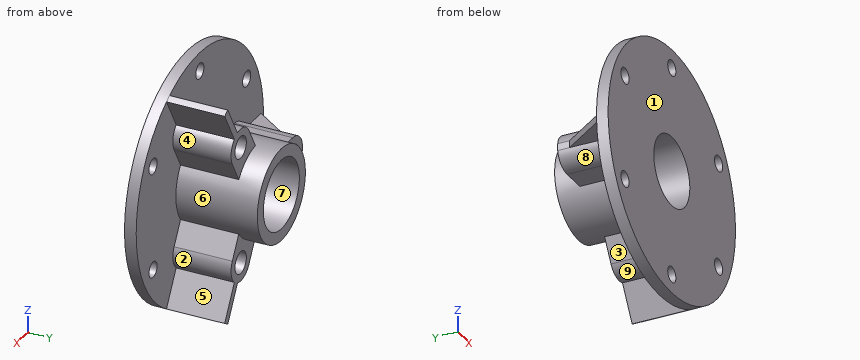
```python
from build123d import *
from build123d.topology import SkipClean

# Parameters (mm, degrees)
SKETCH1_R           = 53
BOSS_EXTRUDE1_DEPTH = 5
SKETCH2_R           = 20
BOSS_EXTRUDE2_DEPTH = 35
SKETCH3_R           = 15
CUT_EXTRUDE1_DEPTH  = 85.958813551
BOSS_EXTRUDE3_START = -25
SKETCH4_R           = 4.75
BOSS_EXTRUDE3_DEPTH = 25
CUT_EXTRUDE2_DEPTH  = 86.902561079
CIRPATTERN1_COUNT   = 3
SKETCH6_R           = 3.4
CUT_EXTRUDE3_DEPTH  = 83.722427431


with BuildPart() as part:
    # Sketch1 → Boss-Extrude1 (new body)
    with BuildSketch(Plane(origin=(0, 0, 0), x_dir=(1, 0, 0), z_dir=(0, 1, 0))):
        with Locations(Location((0, 0, 0), (0, 0, 270))):
            Circle(SKETCH1_R)
    extrude(amount=BOSS_EXTRUDE1_DEPTH)

    # Sketch2 → Boss-Extrude2 (add)
    with BuildSketch(Plane(origin=(0, 5, 0), x_dir=(1, 0, 0), z_dir=(0, 1, 0))):
        with Locations(Location((0, 0, 0), (0, 0, 270))):
            Circle(SKETCH2_R)
    extrude(amount=BOSS_EXTRUDE2_DEPTH)

    # Sketch3 → Cut-Extrude1 (cut, through all)
    with BuildSketch(Plane(origin=(0, 40, 0), x_dir=(1, 0, 0), z_dir=(0, 1, 0))):
        with Locations(Location((0, 0, 0), (0, 0, 270))):
            Circle(SKETCH3_R)
    extrude(amount=-CUT_EXTRUDE1_DEPTH, mode=Mode.SUBTRACT)

    # Sketch4 → Boss-Extrude3 (add)
    with BuildSketch(Plane(origin=(0, 30, 0), x_dir=(1, 0, 0), z_dir=(0, 1, 0)).offset(BOSS_EXTRUDE3_START)):
        with BuildLine():
            Line((-29, 8), (-18.33030278, 8))
            ThreePointArc((-18.33030278, 8), (-20, 0), (-18.33030278, -8))
            Line((-18.33030278, -8), (-29, -8))
            ThreePointArc((-29, -8), (-34.099019514, -6.164414003), (-36.858116823, -1.5))
            Line((-36.858116823, -1.5), (-52.978769333, -1.5))
            ThreePointArc((-52.978769333, -1.5), (-53, 0), (-52.978769333, 1.5))
            Line((-52.978769333, 1.5), (-36.858116823, 1.5))
            ThreePointArc((-36.858116823, 1.5), (-34.099019514, 6.164414003), (-29, 8))
        make_face()
        with Locations(Location((-29, 0, 0), (0, 0, 270))):
            Circle(SKETCH4_R, mode=Mode.SUBTRACT)
    boss_extrude3 = extrude(amount=BOSS_EXTRUDE3_DEPTH)

    # Sketch5 → Cut-Extrude2 (cut, through all)
    with BuildSketch(Plane.XY.offset(1.5)):
        Polygon((-36.858116823, 25), (-50.978769333, 5), (-53.978769333, 5), (-53.978769333, 30), (-36.858116823, 30), align=None)
    extrude(amount=-CUT_EXTRUDE2_DEPTH, mode=Mode.SUBTRACT)

    # CirPattern1: Boss-Extrude3 ×3 about axis
    with SkipClean():  # the faces are left unmerged after this step: merging them gives an invalid solid
        cirpattern1_axis = Axis((0, 0, 0), (0, 1, 0))
        for i in range(1, CIRPATTERN1_COUNT):
            add(boss_extrude3.rotate(cirpattern1_axis, i * 360 / CIRPATTERN1_COUNT))

    # Sketch6 → Cut-Extrude3 (cut, through all)
    with SkipClean():  # the faces are left unmerged after this step: merging them gives an invalid solid
        with BuildSketch(Plane(origin=(0, 5, 0), x_dir=(1, 0, 0), z_dir=(0, 1, 0))):
            with Locations(Location((0, 45, 0), (0, 0, 270))):
                Circle(SKETCH6_R)
            with Locations(Location((38.97114317, 22.5, 0), (0, 0, 270))):
                Circle(SKETCH6_R)
            with Locations(Location((38.97114317, -22.5, 0), (0, 0, 270))):
                Circle(SKETCH6_R)
            with Locations(Location((0, -45, 0), (0, 0, 270))):
                Circle(SKETCH6_R)
            with Locations(Location((-38.97114317, -22.5, 0), (0, 0, 270))):
                Circle(SKETCH6_R)
            with Locations(Location((-38.97114317, 22.5, 0), (0, 0, 270))):
                Circle(SKETCH6_R)
        extrude(amount=-CUT_EXTRUDE3_DEPTH, mode=Mode.SUBTRACT)


solid = part.part
```
Design review of the part built by this model. Coordinates are the model's own, in mm. Face numbers are marked on the shaded views. A direction names the side the tool comes from. Round coordinates to 2 decimals unless told otherwise and drop trailing zeros. Write each loop counter-clockwise with the first axis right and the second up, starting at its lowest first coordinate (ties: lowest second). Pieces come first, ordered by that corner, then holes.
Item 1: We need section D-D on y = 34.5. Write out the cut boundary in (x, z).
Item 2: We need section B-B on x = 0. Write out the cut boundary in (y, z).
Item 3: For probe 1 along X at (y, z) = (4, 20.5); probe 2 along X at (y, z) = (1, -22.5); probe 3 along Y at (x, z) = (-38.5, -10), list the stretches that pass through material, from the lowest coordinate up.
Item 4: We need section A-A on z = 0. Write out the cut boundary in (x, y), and give its area (3 significant figures).
Item 5: Clearance check with flat-ended pins moving along their axes: pin 1 Ø1.5 at (x, y) = (-5.5, 28) entering from -Z; pin 2 Ø3 at (x, y) = (-22.5, 17.5) entering from +Z; pin 3 Ø1.5 at (y, z) = (33.5, -9) entering from -X. State where each tip first meets the part, or that it passes through.
Item 6: The part is to be moulded in two halves that separate along Z. For the marked faces 1, 2, 3 and 4, say which applies: +Z half, -Z half, draft (parallel to the pull), parting line (faces both ways), or undercut.
Item 7: We need section C-C on y = 28.5. Write out the cut boundary in (x, z), and give its area (3 significant figures).
Item 8: For the marked faces 5, 6, 7, 8 and 9, list the 3-axis set-ups (+Z, -Z, +X, -X, +Y, -Y) from which the entire face can be reached by the end or side of a thin tool; tool diameter is ignored.
Returned:
1. outline: circle Ø40 at (0, 0); hole circle Ø30 at (0, 0)
2. outline: (0, -53) - (5, -53) - (5, -48.4) - (0, -48.4) - close; (0, -41.6) - (5, -41.6) - (5, -20) - (40, -20) - (40, -15) - (0, -15) - close; (0, 15) - (40, 15) - (40, 20) - (5, 20) - (5, 41.6) - (0, 41.6) - close; (0, 48.4) - (5, 48.4) - (5, 53) - (0, 53) - close
3. probe 1: x = -48.87 to -41.72, -36.22 to 36.22, 41.72 to 48.87
3. probe 2: x = -47.99 to -42.37, -35.57 to 35.57, 42.37 to 47.99
3. probe 3: y = 0 to 5
4. outline: (-53, 0) - (-15, 0) - (-15, 40) - (-20, 40) - (-20, 30) - (-24.25, 30) - (-24.25, 5) - (-33.75, 5) - (-33.75, 30) - (-36.86, 30) - (-36.86, 25) - (-50.98, 5) - (-53, 5) - close; (15, 0) - (53, 0) - (53, 5) - (20, 5) - (20, 40) - (15, 40) - close
4. area: 1,060 mm2
5. pin 1: stops at z = -19.43
5. pin 2: stops at z = 8
5. pin 3: stops at x = -18.22
6. face 1: draft
6. face 2: undercut
6. face 3: -Z half
6. face 4: undercut
7. outline: (-36.86, -1.5) arc R8 ccw to (-29, -8) - (-18.33, -8) arc R20 ccw to (2.24, -19.87) - (7.57, -29.11) arc R8 ccw to (17.13, -32.67) - (25.19, -46.63) arc R53 ccw to (27.79, -45.13) - (19.73, -31.17) arc R8 ccw to (21.43, -21.11) - (16.09, -11.87) arc R20 ccw to (16.09, 11.87) - (21.43, 21.11) arc R8 ccw to (19.73, 31.17) - (27.79, 45.13) arc R53 ccw to (25.19, 46.63) - (17.13, 32.67) arc R8 ccw to (7.57, 29.11) - (2.24, 19.87) arc R20 ccw to (-18.33, 8) - (-29, 8) arc R8 ccw to (-36.86, 1.5) - close; hole circle Ø9.5 at (-29, 0); hole circle Ø30 at (0, 0); hole circle Ø9.5 at (14.5, -25.11); hole circle Ø9.5 at (14.5, 25.11)
7. area: 1,190 mm2
8. face 5: +X, +Y
8. face 6: +Y
8. face 7: +Y, -Y
8. face 8: -Z, -X, +Y
8. face 9: -Z, +Y
